Can you work these out from the model? Positions are in its coordinate system, mm. A direction names the side the tool comes from. Coordinates: 2 decimals unless noted, no trailing zeros. Order: outer loops, then holes, each group sorted by start corner. A loop starts at its lowest first (then second) coordinate and runs counter-clockwise, first axis right, second up. Notation, with made-up numbers: M 39,8.5 L 56,8.5 A27 ccw 56,35.5 Z; hole C -11.5,8.25 d2. An arc over 180 degrees is marked long. Answer as a JSON object with one key per item and string values.
from build123d import *

# Parameters (mm, degrees)
SKETCH2_W                                           = 540
SKETCH2_H                                           = 150
BOSS_EXTRUDE1_DEPTH                                 = 30
SKETCH3_W                                           = 540
SKETCH3_H                                           = 30
BOSS_EXTRUDE2_DEPTH                                 = 80
SKETCH6_R                                           = 28.5
CUT_EXTRUDE1_DEPTH                                  = 313.769883461
CHAMFER1_SIZE                                       = 2
M30X2_0_TAPPED_HOLE1_D                              = 28
CBORE_FOR_M8_HEX_SOCKET_HEAD_CAP_SCREW1_D           = 8.4
CBORE_FOR_M8_HEX_SOCKET_HEAD_CAP_SCREW1_CBORE_D     = 15
CBORE_FOR_M8_HEX_SOCKET_HEAD_CAP_SCREW1_CBORE_DEPTH = 8.6


with BuildPart() as part:
    # Sketch2 → Boss-Extrude1 (new body)
    with BuildSketch(Plane(origin=(0, 0, 0), x_dir=(1, 0, 0), z_dir=(0, 1, 0))):
        Rectangle(SKETCH2_W, SKETCH2_H)
    extrude(amount=BOSS_EXTRUDE1_DEPTH)

    # Sketch3 → Boss-Extrude2 (add)
    with BuildSketch(Plane(origin=(0, 0, -75), x_dir=(-1, 0, 0), z_dir=(0, 0, -1))):
        with Locations((0, 15)):
            Rectangle(SKETCH3_W, SKETCH3_H)
    extrude(amount=BOSS_EXTRUDE2_DEPTH)

    # Sketch6 → Cut-Extrude1 (cut, through all)
    with BuildSketch(Plane(origin=(0, 0, 0), x_dir=(-1, 0, 0), z_dir=(0, -1, 0))):
        with Locations(Location((-216, 115, 0), (0, 0, 90))):
            Circle(SKETCH6_R)
    cut_extrude1 = extrude(amount=-CUT_EXTRUDE1_DEPTH, mode=Mode.SUBTRACT)

    # Mirror1: Cut-Extrude1 across plane
    add(cut_extrude1.mirror(Plane(origin=(0, 0, 0), x_dir=(0, 0, 1), z_dir=(1, 0, 0))), mode=Mode.SUBTRACT)

    # Chamfer1
    chamfer1_edges = [part.edges().sort_by_distance(p)[0] for p in [
        (-270, 30, -40),
        (0, 30, -155),
        (270, 15, -155),
        (0, 0, -155),
        (0, 30, 75),
        (-270, 15, -155),
        (270, 30, -40),
        (0, 0, 75),
        (-270, 0, -40),
        (270, 0, -40),
        (270, 15, 75),
        (-270, 15, 75),
    ]]
    chamfer(chamfer1_edges, length=CHAMFER1_SIZE)

    # M30x2.0 Tapped Hole1 (through all)
    with Locations(Plane(origin=(0, 30, 0), x_dir=(1, 0, 0), z_dir=(0, 1, 0))):
        with Locations((0, 0)):
            Hole(M30X2_0_TAPPED_HOLE1_D / 2)

    # CBORE for M8 Hex Socket Head Cap Screw1 (through all)
    with Locations(Plane(origin=(0, 30, 0), x_dir=(1, 0, 0), z_dir=(0, 1, 0))):
        with Locations((-238.5, 17.5), (-218.5, 17.5), (-238.5, -17.5), (-218.5, -17.5), (218.5, 18.7), (238.5, 18.7), (218.5, -16.3), (238.5, -16.3)):
            CounterBoreHole(CBORE_FOR_M8_HEX_SOCKET_HEAD_CAP_SCREW1_D / 2, CBORE_FOR_M8_HEX_SOCKET_HEAD_CAP_SCREW1_CBORE_D / 2, CBORE_FOR_M8_HEX_SOCKET_HEAD_CAP_SCREW1_CBORE_DEPTH)


solid = part.part
Item 1: If we mould it in two halves opening along Z, with no side actions, what happens to faces 3 (the flat face through (4, 30, -38)), 4 (the cylindrical face through (-224, 25.8, -22.6)), 5 (the flat face through (-4, 15, 75))? For each: pulls with the +Z half, pulls with the -Z half, needs draft (parallel to the pull), parting line crosses it, or undercut.
Answers follow:
{"face 3": "needs draft", "face 4": "undercut", "face 5": "pulls with the +Z half"}
Item 2: Please list where these lines run through material, in increasing order: line 1 (Z direction, x = -218.5, y = 10.25); line 2 (X direction, y = 17.5, z = -96.5); line 3 (Z direction, x = -218, y = 25).
Answers follow:
{"line 1": "z = -155 to -143.39, -86.61 to -21.7, -13.3 to 13.3, 21.7 to 75", "line 2": "x = -270 to -237.68, -194.32 to 194.32, 237.68 to 270", "line 3": "z = -155 to -143.43, -86.57 to -24.98, -10.02 to 10.02, 24.98 to 75"}
Item 3: I want a section at D-D, the plane z = -115. Write out the boundary of the cut face in (x, y), plus the area to 3 significant figures.
Answers follow:
{"outline": "M -270,2 L -268,0 L -244.5,0 L -244.5,30 L -268,30 L -270,28 Z; M -187.5,0 L 187.5,0 L 187.5,30 L -187.5,30 Z; M 244.5,0 L 268,0 L 270,2 L 270,28 L 268,30 L 244.5,30 Z", "area": "12,800 mm^2"}
Item 4: I'm going to push flat-ended pins straight in: pin 1 (4.5 mm diameter, centred on x = -220.5, z = -16, fed in from +Y); pin 2 (4.5 mm diameter, centred on x = 219.5, z = 16, fed in from +Y) (1 decimal). Where does each tip first touch, or does it pass through?
Answers follow:
{"pin 1": "stops at y = 21.4", "pin 2": "passes through"}
Item 5: Which directions (+Z, -Z, +X, -X, +Y, -Y) give clear straight access to the entire face, cutting with the end or side of a thin tool? Please do faces 1 (the cylindrical face through (-12.932, 14.79, 5.362)), 2 (the flat face through (-215, 21.4, -14)).
Answers follow:
{"face 1": "+Y, -Y", "face 2": "+Y"}
Item 6: I want a section at C-C, the plane y = 10.5. Give the number of separate pieces and of enclosed holes in the cut face, plus the area to 3 significant figures.
Answers follow:
{"separate pieces": "1", "enclosed holes": "11", "area": "118,000 mm^2"}
Item 7: I want a section at A-A, the plane x = 0. Write out the boundary of the cut face in (y, z), plus the area to 3 significant figures.
Answers follow:
{"outline": "M 0,-153 L 2,-155 L 28,-155 L 30,-153 L 30,-14 L 0,-14 Z; M 0,14 L 30,14 L 30,73 L 28,75 L 2,75 L 0,73 Z", "area": "6,050 mm^2"}
Item 8: I want a section at B-B, the plane z = 0. Write out the boundary of the cut face in (x, y).
Answers follow:
{"outline": "M -270,2 L -268,0 L -14,0 L -14,30 L -268,30 L -270,28 Z; M 14,0 L 268,0 L 270,2 L 270,28 L 268,30 L 14,30 Z"}
